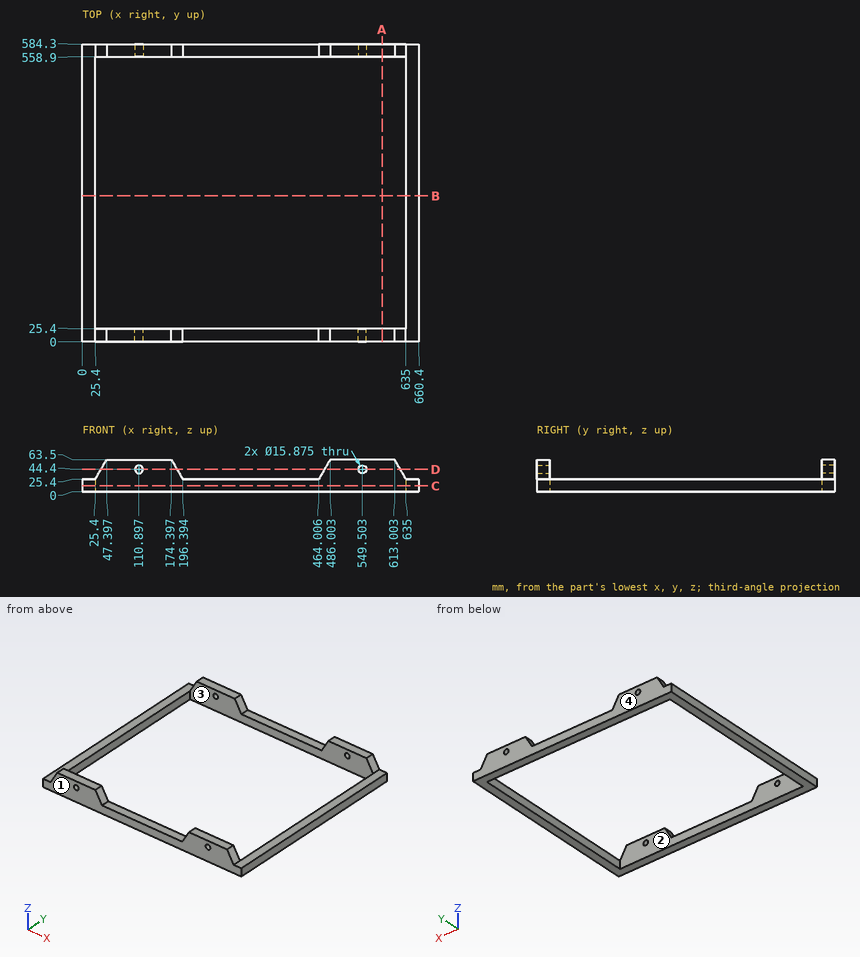
Drawing for the job (mm, zero at the part's lowest x, y, z). A direction names the side the tool comes from. Coordinates: 2 decimals unless noted, no trailing zeros. Order: outer loops, then holes, each group sorted by start corner. A loop starts at its lowest first (then second) coordinate and runs counter-clockwise, first axis right, second up.
Item 1: Pin check, flat tips, straight feed: pin 1 Ø12.5 at (x, z) = (110.9, 44.4) entering from -Y; pin 2 Ø12.5 at (x, y) = (8.5, 254) entering from +Z; pin 3 Ø19 at (x, z) = (344.5, 26) entering from -Y. Stop position of each tip, or through.
Check sheet entries:
pin 1: passes through
pin 2: stops at z = 25.4
pin 3: stops at y = 0
Item 2: Two-plate mould, pull along X, no slides. Class the marked faces 1 and 2: +X half, -X half, draft (parallel to the pull), parting line (faces both ways), or undercut.
Check sheet entries:
face 1: draft
face 2: undercut
Item 3: Band-saw the part on C-C on z = 12. List the corners of the cut face in (x, y).
Check sheet entries:
outline: (0, 0) - (660.4, 0) - (660.4, 584.3) - (0, 584.3) - close; hole (25.4, 25.4) - (635, 25.4) - (635, 558.9) - (25.4, 558.9) - close
Item 4: 3-axis set-ups, long thin cutter, end or side, ignore diameter. For the marked faces 3 and 4: which of +Z, -Z, +X, -X, +Y, -Y reach the whole face in a straight line?
Check sheet entries:
face 3: +Z, -Z
face 4: +Z, -Z, +X, -X, +Y
Item 5: Band-saw the part on A-A on x = 588. List the corners of the cut face in (y, z).
Check sheet entries:
outline: (0, 0) - (25.4, 0) - (25.4, 63.5) - (0, 63.5) - close; (558.9, 0) - (584.3, 0) - (584.3, 63.5) - (558.9, 63.5) - close
Item 6: Band-saw the part on B-B on y = 286. List the corners of the cut face in (x, z), plus the area to 3 significant figures.
Check sheet entries:
outline: (0, 0) - (25.4, 0) - (25.4, 25.4) - (0, 25.4) - close; (635, 0) - (660.4, 0) - (660.4, 25.4) - (635, 25.4) - close
area: 1,290 mm2
Item 7: Drill centre lines: L1, parallel to Y at x = 72, z = 11.5; L2, parallel to X at y = 170, z = 8.5; L3, parallel to X at y = 19, z = 44 (1 decimal). Where is each one in solid material? Low to high.
Check sheet entries:
L1: y = 0 to 25.4, 558.9 to 584.3
L2: x = 0 to 25.4, 635 to 660.4
L3: x = 36.1 to 103, 118.8 to 185.7, 474.7 to 541.6, 557.4 to 624.3
Item 8: Band-saw the part on D-D on z = 44.4. Give the number of separate pieces and of enclosed holes in the cut face, plus the area to 3 significant figures.
Check sheet entries:
separate pieces: 8
enclosed holes: 0
area: 13,500 mm2
